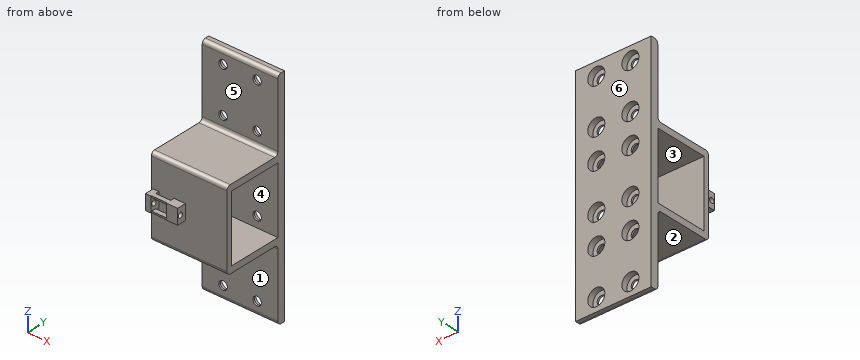
from build123d import *

# Parameters (mm, degrees)
SKETCH1_W                                        = 35.2
SKETCH1_H                                        = 28.2
BOSS_EXTRUDE1_DEPTH                              = 40
FILLET1_R                                        = 2
CBORE_FOR_M4_PAN_HEAD_MACHINE_SCREW1_D           = 4.5
CBORE_FOR_M4_PAN_HEAD_MACHINE_SCREW1_DEPTH       = 4
CBORE_FOR_M4_PAN_HEAD_MACHINE_SCREW1_CBORE_D     = 9
CBORE_FOR_M4_PAN_HEAD_MACHINE_SCREW1_CBORE_DEPTH = 3.1
SKETCH5_W                                        = 8
SKETCH5_H                                        = 4.7
SKETCH5_R                                        = 1.35
BOSS_EXTRUDE2_DEPTH                              = 3
SKETCH6_W                                        = 8
SKETCH6_H                                        = 4.7
SKETCH6_R                                        = 1.35
BOSS_EXTRUDE3_DEPTH                              = 6
BOSS_EXTRUDE4_REACH                              = 129.609
SKETCH7_W                                        = 0.8
SKETCH7_H                                        = 2.4
SKETCH8_W                                        = 0.8
SKETCH8_H                                        = 2.4
BOSS_EXTRUDE5_DEPTH                              = 2


with BuildPart() as part:
    # Sketch1 → Boss-Extrude1 (new body)
    with BuildSketch(Plane(origin=(0, 0, 0), x_dir=(0, 0, -1), z_dir=(1, 0, 0))):
        Polygon((0, 0), (118, 0), (118, -4), (80, -4), (80, -35), (38, -35), (38, -4), (0, -4), align=None)
        with Locations((59, -18.1)):
            Rectangle(SKETCH1_W, SKETCH1_H, mode=Mode.SUBTRACT)
    extrude(amount=-BOSS_EXTRUDE1_DEPTH)

    # Fillet1
    fillet1_edges = [part.edges().sort_by_distance(p)[0] for p in [
        (-20, -4, -118),
        (-20, -4, -80),
        (-20, -35, -80),
        (-20, -35, -38),
        (-20, -4, -38),
        (-20, -4, 0),
    ]]
    fillet(fillet1_edges, radius=FILLET1_R)

    # CBORE for M4 Pan Head Machine Screw1
    with Locations(Plane(origin=(-11, 0, -111), x_dir=(0, 0, 1), z_dir=(0, 1, 0))):
        with Locations((0, 0), (0, -18), (24, 0), (24, -18), (40, 0), (64, 0), (64, -18), (40, -18), (80, 0), (80, -18), (104, -18), (104, 0)):
            CounterBoreHole(CBORE_FOR_M4_PAN_HEAD_MACHINE_SCREW1_D / 2, CBORE_FOR_M4_PAN_HEAD_MACHINE_SCREW1_CBORE_D / 2, CBORE_FOR_M4_PAN_HEAD_MACHINE_SCREW1_CBORE_DEPTH, depth=CBORE_FOR_M4_PAN_HEAD_MACHINE_SCREW1_DEPTH)

    # Sketch5 → Boss-Extrude2 (add)
    with BuildSketch(Plane(origin=(-39, 0, 0), x_dir=(0, 0, -1), z_dir=(1, 0, 0))):
        with Locations((59, -37.35)):
            Rectangle(SKETCH5_W, SKETCH5_H)
        with Locations((59, -38)):
            Circle(SKETCH5_R, mode=Mode.SUBTRACT)
    extrude(amount=BOSS_EXTRUDE2_DEPTH)

    # Sketch6 → Boss-Extrude3 (add)
    with BuildSketch(Plane(origin=(-28, 0, 0), x_dir=(0, 0, -1), z_dir=(1, 0, 0))):
        with Locations((59, -37.35)):
            Rectangle(SKETCH6_W, SKETCH6_H)
        with Locations((59, -38)):
            Circle(SKETCH6_R, mode=Mode.SUBTRACT)
    extrude(amount=BOSS_EXTRUDE3_DEPTH)

    # Sketch7 → Boss-Extrude4 (add, up to next)
    with BuildSketch(Plane.ZY.offset(28), mode=Mode.PRIVATE) as boss_extrude4_sk1:
        with Locations((-62.6, -38.2)):
            Rectangle(SKETCH7_W, SKETCH7_H)
    boss_extrude4_tool1 = extrude(boss_extrude4_sk1.sketch, amount=BOSS_EXTRUDE4_REACH, mode=Mode.PRIVATE) - part.part
    # Sketch7 → Boss-Extrude4 (add, up to next)
    with BuildSketch(Plane.ZY.offset(28), mode=Mode.PRIVATE) as boss_extrude4_sk2:
        with Locations((-55.4, -38.2)):
            Rectangle(SKETCH7_W, SKETCH7_H)
    boss_extrude4_tool2 = extrude(boss_extrude4_sk2.sketch, amount=BOSS_EXTRUDE4_REACH, mode=Mode.PRIVATE) - part.part
    add(boss_extrude4_tool1.solids().sort_by_distance((-28, -38.2, -62.6))[0])
    add(boss_extrude4_tool2.solids().sort_by_distance((-28, -38.2, -55.4))[0])

    # Sketch8 → Boss-Extrude5 (add)
    with BuildSketch(Plane(origin=(-36, 0, 0), x_dir=(0, 0, -1), z_dir=(1, 0, 0))):
        with Locations((62.6, -38.2)):
            Rectangle(SKETCH8_W, SKETCH8_H)
        with Locations((55.4, -38.2)):
            Rectangle(SKETCH8_W, SKETCH8_H)
    extrude(amount=BOSS_EXTRUDE5_DEPTH)


solid = part.part
For this review, take the finished solid that the model builds, in its own axes (mm). Face numbers are marked on the shaded views. A direction names the side the tool comes from. Coordinates: 2 decimals unless noted, no trailing zeros. Loops run counter-clockwise (first coordinate to the right, second up) from the corner with the lowest first, then second, coordinate; pieces in that order, holes last. Notation, with made-up numbers: (11.25, 53.25) - (27.25, 53.25) arc R12 cw to (27.25, 58.25) - close; hole circle Ø10 at (-30.75, 1.5). An arc over 180 degrees is marked (long way). Use a Markdown table: item, result. Add a question column.
Item 1: We need section A-A (z = -111). Give the boundary of the cut face in (x, y), and give its area (3 significant figures).
Item 2: We need section D-D (z = -86). Give the boundary of the cut face in (x, y), and give its area (3 significant figures).
Item 3: Insertion check: pin 1 Ø10.5 at (x, z) = (-11, -7) entering from -Y; pin 2 Ø5.5 at (x, z) = (-11, -71) entering from -Y; pin 3 Ø10 at (x, y) = (-27.5, -29.5) entering from +Z; pin 4 Ø2.5 at (x, z) = (-11, -7) entering from +Y. Each pin has a flat end and moves straight along its axis. Give the tip position at first contact, or say it passes through.
Item 4: Mouldability with a two-part tool opening along Y and no side actions: class the marked faces 1, 2 and 3 as pulls with the +Y half, pulls with the -Y half, needs draft (parallel to the pull), parting line crosses it, or undercut.
Item 5: For line 1 (X direction, y = -3, z = -47); line 2 (X direction, y = -3.55, z = -7); line 3 (Z direction, x = -25.5, y = -20.5), list the stretches that pass through material, from the lowest coordinate up.
Item 6: We need section B-B (y = -28). Give the boundary of the cut face in (x, z).
Item 7: We need section C-C (z = -13.5). Give the boundary of the cut face in (x, y), and give its area (3 significant figures).
Item 8: Tool access review of the marked faces 4, 5 and 6: name each direction out of +Z, -Z, +X, -X, +Y, -Y from which nothing blocks a thin tool from reaching the whole face with its end or side.
Results list:
| question | item | result |
|---|---|---|
| 1 | outline | (-40, -4) - (-31.25, -4) - (-31.25, -3.1) - (-33.5, -3.1) - (-33.5, 0) - (-40, 0) - close; (-26.75, -4) - (-13.25, -4) - (-13.25, -3.1) - (-15.5, -3.1) - (-15.5, 0) - (-24.5, 0) - (-24.5, -3.1) - (-26.75, -3.1) - close; (-8.75, -4) - (0, -4) - (0, 0) - (-6.5, 0) - (-6.5, -3.1) - (-8.75, -3.1) - close |
| 1 | area | 96.1 mm^2 |
| 2 | outline | (-40, -4) - (-31.02, -4) - (-31.02, -3.1) - (-33.39, -3.1) - (-33.39, 0) - (-40, 0) - close; (-26.98, -4) - (-13.02, -4) - (-13.02, -3.1) - (-15.39, -3.1) - (-15.39, 0) - (-24.61, 0) - (-24.61, -3.1) - (-26.98, -3.1) - close; (-8.98, -4) - (0, -4) - (0, 0) - (-6.61, 0) - (-6.61, -3.1) - (-8.98, -3.1) - close |
| 2 | area | 98.3 mm^2 |
| 3 | pin 1 | stops at y = -4 |
| 3 | pin 2 | stops at y = -35 |
| 3 | pin 3 | stops at z = -38 |
| 3 | pin 4 | passes through |
| 4 | face 1 | pulls with the -Y half |
| 4 | face 2 | needs draft |
| 4 | face 3 | undercut |
| 5 | line 1 | x = -40 to -33.5, -24.5 to -15.5, -6.5 to 0 |
| 5 | line 2 | x = -40 to -31.25, -26.75 to -13.25, -8.75 to 0 |
| 5 | line 3 | z = -80 to -76.6, -41.4 to -38 |
| 6 | outline | (-40, -80) - (0, -80) - (0, -76.6) - (-40, -76.6) - close; (-40, -41.4) - (0, -41.4) - (0, -38) - (-40, -38) - close |
| 7 | outline | (-40, -4) - (0, -4) - (0, 0) - (-40, 0) - close |
| 7 | area | 160 mm^2 |
| 8 | face 4 | +X, -X |
| 8 | face 5 | +Z, +X, -X, -Y |
| 8 | face 6 | +Z, -Z, +X, -X, +Y |
